Verification items for the finished model (mm, model axes). A direction names the side the tool comes from. Coordinates: 2 decimals unless noted, no trailing zeros. Order: outer loops, then holes, each group sorted by start corner. A loop starts at its lowest first (then second) coordinate and runs counter-clockwise, first axis right, second up. Notation, with made-up numbers: M -23.75,42 L -5.75,42 A9 cw -5.75,55 Z; hole C -9.5,29.25 d5. An arc over 180 degrees is marked long. Return JSON: item names as keys, results as strings. Group by question number.
1. Section check B-B, the plane y = 52. Record the cut outline in (x, z).
2. Gauge pin test, flat ends, axial feed: pin 1 (12 mm diameter, centred on y = -4, z = -21, fed in from +X); pin 2 (4 mm diameter, centred on y = 11, z = -5, fed in from -X); pin 3 (1.5 mm diameter, centred on x = -49, z = -17, fed in from +Y); pin 4 (1 mm diameter, centred on y = -31, z = -22, fed in from +X). Record the tip position at first contact, or that the pin passes through.
3. Set-up check for faces 4 (the cylindrical face through (-3.64, 47.31, -0.77)), 5 (the cylindrical face through (62.5, 57.15, -1.22)): record each of +Z, -Z, +X, -X, +Y, -Y from which the full face is reachable in a straight line by a thin tool's end or side.
4. Mould release check, pull along Y, two halves, no side actions. Record for faces 1 (the flat face through (-36.084, -35, 0)), 2 (the flat face through (61, 70.462, 0)), 3 (the cylindrical face through (-68.086, 6.05, 0.088)): +Y half, -Y half, draft (parallel to the pull), parting line (faces both ways), or undercut.
5. Section check A-A, the plane z = 0. Record the cut outline in (x, y), plus the area to 3 significant figures.
6. Section check C-C, the plane x = -5. Record the cut outline in (y, z).
7. Material ranges on line 1 along X through (y, z) = (-29.5, 3); line 2 along Y through (x, z) = (-47, 21.5); line 3 along X through (y, z) = (-64, -11), recorded low to high.
Autodesk Inventor part; units mm, degrees
ref_plane "YZ Plane" through (0, 0, 0) normal (1, 0, 0) x (0, 1, 0)
ref_plane "XZ Plane" through (0, 0, 0) normal (0, 1, 0) x (-1, 0, 0)
ref_plane "XY Plane" through (0, 0, 0) normal (0, 0, 1) x (1, 0, 0)
ref_plane "Work Plane1" through (-36.0844, -34.5379, 0) normal (-1, 0, 0) x (0, -1, 0)
sketch "Sketch1" plane through (-36.0844, -34.5379, 0) normal (-1, 0, 0) x (0, -1, 0)
  circle A0 centre (0, 0) radius 37.75
  point P0 (-34.5379, 0)
  dimension "d4" = 75.5
extrude "Extrusion1" add sketch "Sketch1" along normal blind 26.5
fillet "Fillet1" radius 9 2 edges at (-62.5844, 3.2121, 0) (-36.0844, 3.2121, 0)
sketch "Sketch2" plane through (-36.0844, -34.5379, 0) normal (-1, 0, 0) x (0, -1, 0)
  circle A0 centre (0, 0) radius 2
  point P0 (-34.5379, 0)
  dimension "d8" = 4
sketch3d "3D Sketch1"
  line L0 (-36.0844, -34.5379, 0) -> (-70.0844, -34.5379, 0)
  line L1 (-70.0844, -34.5379, 0) -> (-70.0844, 45.4621, 0)
  line L2 (-70.0844, 45.4621, 0) -> (60.9156, 45.4621, 0)
  line L3 (60.9156, 45.4621, 0) -> (60.9156, 70.4621, 0)
  dimension "d0" = 34
  dimension "d1" = 80
  dimension "d2" = 131
  dimension "d3" = 25
sweep "Sweep1" add profiles "Sketch2" path "3D Sketch1"
properties part number "Main Landing Gear"
Answers follow:
{
 "1": {"outline": "C 60.92,0 d4"},
 "2": {"pin 1": "x = -36.39", "pin 2": "through", "pin 3": "y = -0.46", "pin 4": "x = -36.08"},
 "3": {"face 4": "none", "face 5": "+Y"},
 "4": {"face 1": "draft", "face 2": "+Y half", "face 3": "undercut"},
 "5": {"outline": "M -72.08,-36.54 L -62.58,-36.54 L -62.58,-63.29 A9 ccw -53.58,-72.29 L -45.08,-72.29 A9 ccw -36.08,-63.29 L -36.08,-5.79 A9 ccw -45.08,3.21 L -53.58,3.21 A9 ccw -62.58,-5.79 L -62.58,-32.54 L -68.08,-32.54 L -68.08,43.46 L 62.92,43.46 L 62.92,70.46 L 58.92,70.46 L 58.92,47.46 L -72.08,47.46 Z", "area": "2,910 mm^2"},
 "6": {"outline": "C 45.46,0 d4"},
 "7": {"line 1": "-62.58 to -36.08", "line 2": "-65.57 to -3.51", "line 3": "-62.17 to -36.5"}
}
